from build123d import *

# Parameters (mm, degrees)
F0_R     = 6.35
F1_DEPTH = 80.8482
F2_R     = 6.35
F2_R_2   = 3.175
F3_DEPTH = 12.7
F4_R     = 2.7559
F5_DEPTH = 12.7
F6_R     = 2.7559
F7_DEPTH = 2.54
F7_TAPER = 45


with BuildPart() as f1:
    # F0 (on Front) → F1 (new body)
    with BuildSketch(Plane.XZ):
        Circle(F0_R)
    extrude(amount=F1_DEPTH)

    # F2 (on face) → F3 (cut)
    with BuildSketch(Plane.XZ.offset(80.8482)):
        Circle(F2_R)
        Circle(F2_R_2, mode=Mode.SUBTRACT)
    extrude(amount=-F3_DEPTH, mode=Mode.SUBTRACT)

    # F4 (on face) → F5 (cut)
    with BuildSketch(Plane(origin=(0, 0, 0), x_dir=(-1, 0, 0), z_dir=(0, 1, 0))):
        Circle(F4_R)
    extrude(amount=-F5_DEPTH, mode=Mode.SUBTRACT)

    # F6 (on face) → F7 (cut)
    with BuildSketch(Plane(origin=(0, -12.7, 0), x_dir=(-1, 0, 0), z_dir=(0, 1, 0))):
        Circle(F6_R)
    extrude(amount=-F7_DEPTH, taper=F7_TAPER, mode=Mode.SUBTRACT)


solid = f1.part
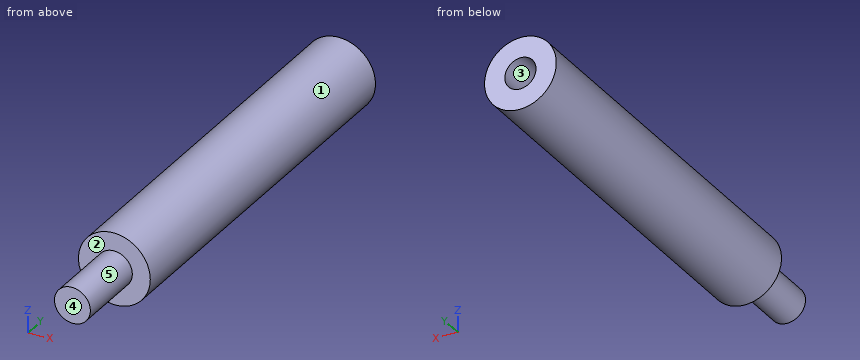
Source: CAD feature listing. Evaluate the final solid. Frame: model axes, mm. Face numbers are marked on the shaded views. A direction names the side the tool comes from. Coordinates: 2 decimals unless noted, no trailing zeros. Order: outer loops, then holes, each group sorted by start corner. A loop starts at its lowest first (then second) coordinate and runs counter-clockwise, first axis right, second up. Notation, with made-up numbers: M -11.75,-12 L 39.25,-12 A20 ccw 39.25,13 Z; hole C 7,12 d8. An arc over 180 degrees is marked long. Write each question's results on one line, items separated by ' | '. Start each with the question number.
1. Draft query along X for the marked faces 1, 2 and 3. Return one class per face: +X half, -X half, draft (parallel to the pull), parting line (faces both ways), or undercut.
2. Section B-B, the plane z = -5.25. Return the cut outline in (x, y), then the cut area to 3 significant figures.
3. Pin query (flat end, axial travel): pin 1 (1 mm diameter, centred on x = 3.5, z = 0, fed in from +Y); pin 2 (4 mm diameter, centred on x = 3.5, y = -58, fed in from -Z); pin 3 (3 mm diameter, centred on x = 3, y = -22, fed in from +Z); pin 4 (2 mm diameter, centred on x = 1.5, z = -4.5, fed in from -Y). Return the tip coordinate at first contact, or that it passes through.
4. Section C-C, the plane x = 4.5. Return the cut outline in (y, z), then the cut area to 3 significant figures.
5. Material intervals for L1, parallel to Z at x = 0, y = -5; L2, parallel to Y at x = 4.5, z = 3.75; L3, parallel to X at y = -42, z = 5.5, sorted ascending.
6. Reachability of the marked faces 4 and 5 from +Z, -Z, +X, -X, +Y, -Y: full face, straight path, thin tool, end or side. Return the list, or none.
7. Section A-A, the plane y = -38.5. Return the cut outline in (x, z).
Solution:
1) face 1: parting line | face 2: draft | face 3: undercut
2) outline: M -3.57,-68.15 L 3.57,-68.15 L 3.57,0 L -3.57,0 Z | area: 487 mm²
3) pin 1: y = 0 | pin 2: z = -6.17 | pin 3: z = 6.17 | pin 4: y = -68.15
4) outline: M -68.15,-4.48 L 0,-4.48 L 0,4.48 L -68.15,4.48 Z | area: 611 mm²
5) L1: -6.35 to -2.76, 2.76 to 6.35 | L2: -68.15 to 0 | L3: -3.17 to 3.17
6) face 4: +Z, -Z, +X, -X, -Y | face 5: -Y
7) outline: C 0,0 d12.7
